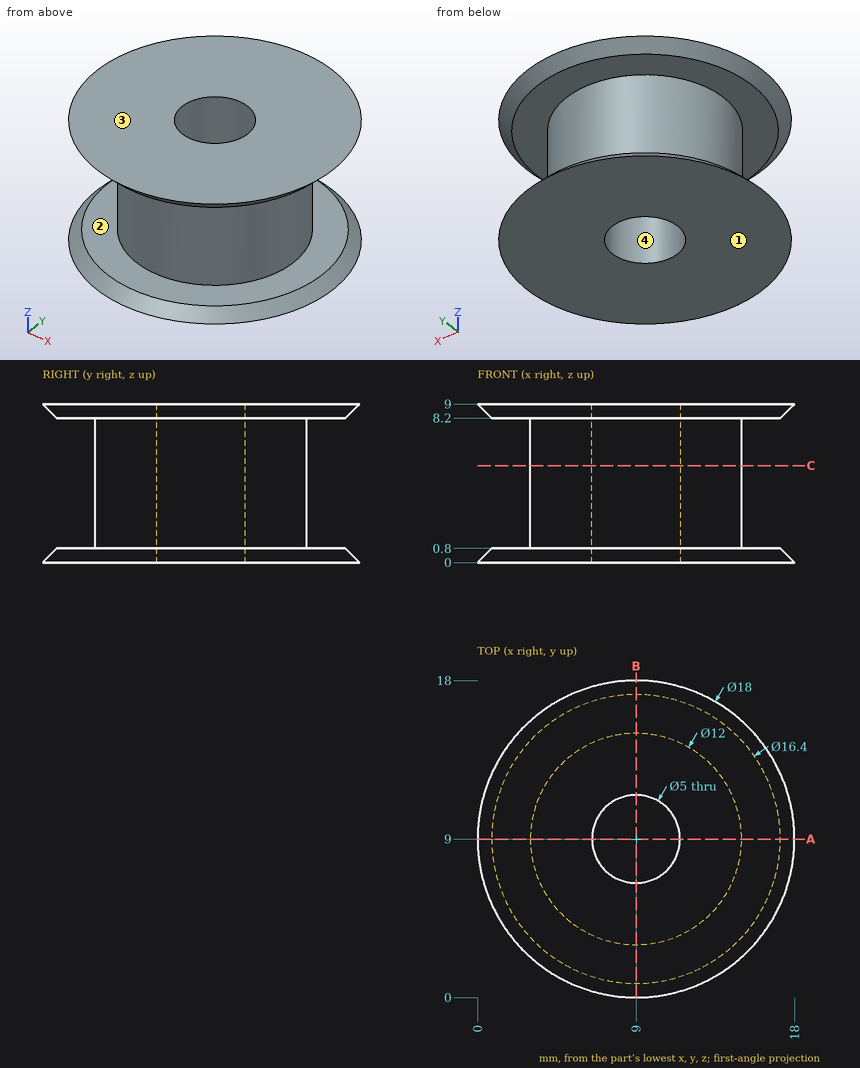
Can you work these out from the drawing? Everything is in mm from the part's minimum corner. Give positions to 0.01 mm unless a question says otherwise; leave off trailing zeros. Write each loop counter-clockwise with the first axis right and the second up, starting at its lowest first coordinate (ties: lowest second). Pieces come first, ordered by that corner, then holes. Notation, with made-up numbers: M -18.75,37.25 L 25.25,37.25 A18 ccw 25.25,57.25 Z; hole C 1,-32 d4. An arc over 180 degrees is marked long. Answer in a Markdown table with one row per item. Add a question column.
Item 1: We'd pull the mould along Z, two halves only. Please class the marked faces 1, 2, 3 and 4: released by +Z, released by -Z, zero draft, split by the parting line, or undercut.
Item 2: Imagine slicing it at C-C, the plane z = 5.5. Write out the boundary of the cut face in (x, y).
Item 3: Imagine slicing it at A-A, the plane y = 9. Write out the boundary of the cut face in (x, z), plus the area to 3 significant figures.
Item 4: For pin 1 Ø4 at (y, z) = (14, 3.5) entering from -X, with a flat end and sliding along its axis, tell me the tip position at first contact or that it passes through.
Item 5: Please list where these lines run through material, in increasing order: L1, parallel to Y at x = 9, z = 4; L2, parallel to Z at x = 16.75, y = 9.5; L3, parallel to Y at x = 10, z = 8.
Evaluation:
| question | item | result |
|---|---|---|
| 1 | face 1 | released by -Z |
| 1 | face 2 | undercut |
| 1 | face 3 | released by +Z |
| 1 | face 4 | zero draft |
| 2 | outline | C 9,9 d12; hole C 9,9 d5 |
| 3 | outline | M 0,0 L 6.5,0 L 6.5,9 L 0,9 L 0.8,8.2 L 3,8.2 L 3,0.8 L 0.8,0.8 Z; M 11.5,0 L 18,0 L 17.2,0.8 L 15,0.8 L 15,8.2 L 17.2,8.2 L 18,9 L 11.5,9 Z |
| 3 | area | 71.3 mm² |
| 4 | pin 1 | stops at x = 3.8 |
| 5 | L1 | y = 3 to 6.5, 11.5 to 15 |
| 5 | L2 | z = 0 to 0.8, 8.2 to 9 |
| 5 | L3 | y = 3.08 to 6.71, 11.29 to 14.92 |
